Geometry check sheet. Reference: drawing and pictorial views, mm from the part's lowest x, y, z. A direction names the side the tool comes from. Give positions to 0.01 mm unless a question says otherwise; leave off trailing zeros. Loops run counter-clockwise (first coordinate to the right, second up) from the corner with the lowest first, then second, coordinate; pieces in that order, holes last. Notation, with made-up numbers: (67.5, -16.75) -> (99.5, -16.75) arc R18 cw to (99.5, 10.25) -> close; hole circle Ø5 at (-32.75, 67.5). An arc over 180 degrees is marked (long way). Write item = value, one per line. Start each with the question number.
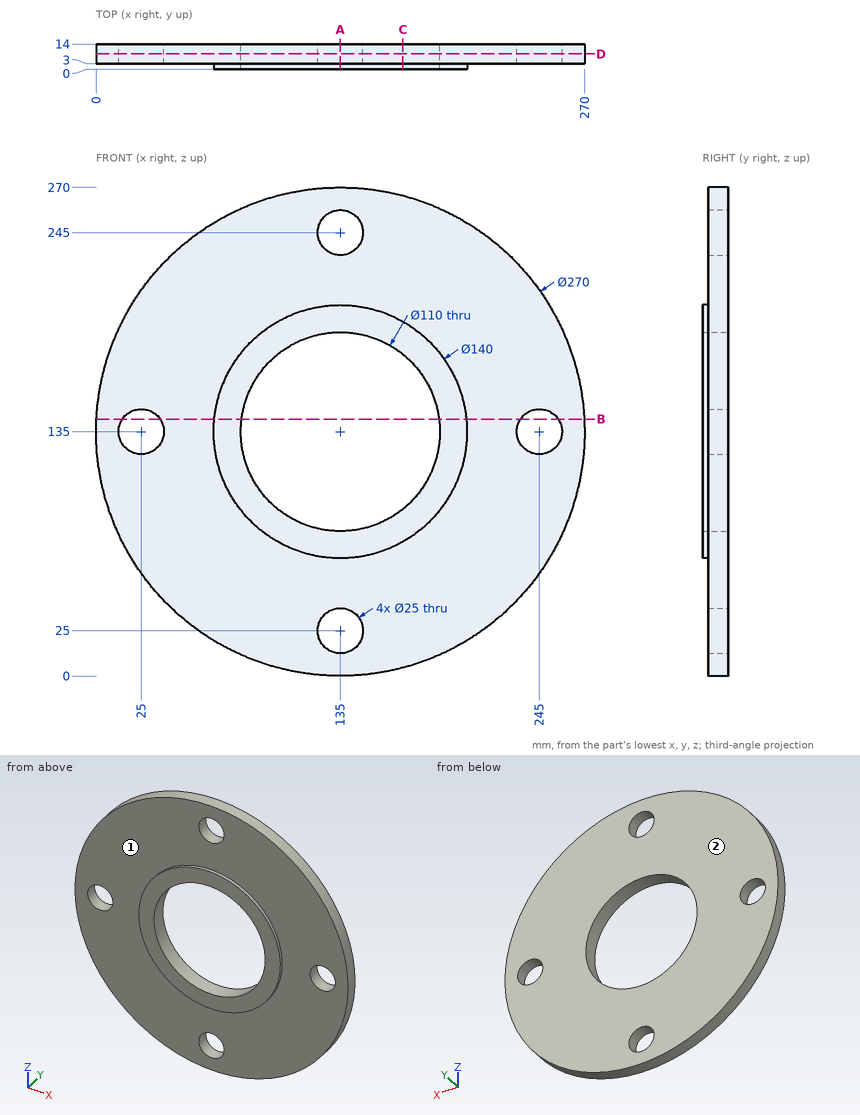
1) Section check D-D (y = 8.5). Enter the section's corners in (x, z), plus the area to 3 significant figures.
2) Section check B-B (z = 142). Enter the section's corners in (x, y).
3) Section check A-A (x = 135). Enter the section's corners in (y, z).
4) Thickness scan on line 1 (X direction, y = 6.25, z = 135); line 2 (Z direction, x = 25, y = 12.25); line 3 (X direction, y = 6.5, z = 91). Record the ranges inside material, lowest first.
5) Depth check by flat-ended pin: pin 1 Ø8 at (x, y) = (193, 12.5) entering from +Z; pin 2 Ø6 at (x, z) = (120, 185.5) entering from +Y; pin 3 Ø8 at (x, y) = (199, 3) entering from +Z; pin 4 Ø12 at (x, z) = (208, 195.5) entering from -Y. Enter the tip coordinate at first touch or a pass-through.
6) Tool access check on the marked faces 1 and 2. Record the directions out of +Z, -Z, +X, -X, +Y, -Y that give a thin tool (end or side, any length) a straight path to the whole face; none if there is none.
7) Section check C-C (x = 169.5). Enter the section's corners in (y, z), plus the area to 3 significant figures.
Check result:
q1.outline = circle Ø270 at (135, 135); hole circle Ø25 at (25, 135); hole circle Ø110 at (135, 135); hole circle Ø25 at (135, 25); hole circle Ø25 at (135, 245); hole circle Ø25 at (245, 135)
q1.area = 45,800 mm2
q2.outline = (0.18, 3) -> (14.64, 3) -> (14.64, 14) -> (0.18, 14) -> close; (35.36, 3) -> (65.35, 3) -> (65.35, 0) -> (80.45, 0) -> (80.45, 14) -> (35.36, 14) -> close; (189.55, 0) -> (204.65, 0) -> (204.65, 3) -> (234.64, 3) -> (234.64, 14) -> (189.55, 14) -> close; (255.36, 3) -> (269.82, 3) -> (269.82, 14) -> (255.36, 14) -> close
q3.outline = (0, 65) -> (3, 65) -> (3, 37.5) -> (14, 37.5) -> (14, 80) -> (0, 80) -> close; (0, 190) -> (14, 190) -> (14, 232.5) -> (3, 232.5) -> (3, 205) -> (0, 205) -> close; (3, 0) -> (14, 0) -> (14, 12.5) -> (3, 12.5) -> close; (3, 257.5) -> (14, 257.5) -> (14, 270) -> (3, 270) -> close
q4.line_1 = 0 to 12.5, 37.5 to 80, 190 to 232.5, 257.5 to 270
q4.line_2 = 56.74 to 122.5, 147.5 to 213.26
q4.line_3 = 7.37 to 102, 168 to 262.63
q5.pin_1 = 258.73
q5.pin_2 = 14
q5.pin_3 = 255.93
q5.pin_4 = 3
q6.face_1 = -Y
q6.face_2 = +Z, -Z, +X, -X, +Y
q7.outline = (0, 74.09) -> (3, 74.09) -> (3, 4.48) -> (14, 4.48) -> (14, 92.17) -> (0, 92.17) -> close; (0, 177.83) -> (14, 177.83) -> (14, 265.52) -> (3, 265.52) -> (3, 195.91) -> (0, 195.91) -> close
q7.area = 2,040 mm2
